from build123d import *

# Parameters (mm, degrees)
ESQUISSE1_W             = 23.5
ESQUISSE1_H             = 23.5
ESQUISSE1_W_2           = 20
ESQUISSE1_H_2           = 20
BOSS_EXTRU_1_DEPTH      = 200
ESQUISSE2_R             = 7.210256751
ENL_V_MAT_EXTRU_1_DEPTH = 1.75


with BuildPart() as part:
    # Esquisse1 → Boss.-Extru.1 (new body)
    with BuildSketch(Plane.XY):
        Rectangle(ESQUISSE1_W, ESQUISSE1_H)
        Rectangle(ESQUISSE1_W_2, ESQUISSE1_H_2, mode=Mode.SUBTRACT)
    extrude(amount=BOSS_EXTRU_1_DEPTH)

    # Esquisse2 → Enlèv. mat.-Extru.1 (cut)
    with BuildSketch(Plane.ZY.offset(11.75)):
        with Locations((100, 0)):
            Circle(ESQUISSE2_R)
    extrude(amount=-ENL_V_MAT_EXTRU_1_DEPTH, mode=Mode.SUBTRACT)


solid = part.part
CAD build for the part. Positions are in the model's coordinates, mm. A direction names the side the tool comes from. Give positions to 0.01 mm unless a question says otherwise; leave off trailing zeros. Write each loop counter-clockwise with the first axis right and the second up, starting at its lowest first coordinate (ties: lowest second). Pieces come first, ordered by that corner, then holes. Notation, with made-up numbers: (18.5, 74) -> (26.5, 74) arc R13 cw to (26.5, 82) -> close; hole circle Ø8 at (-29.75, 42.25). An arc over 180 degrees is marked (long way). Return JSON: item names as keys, results as strings.
Item 1: Tool access for faces 5 (the cylindrical face through (-10.887, 0.317, 92.797)), 6 (the flat face through (10, 0, 99)), 7 (the flat face through (-11, 0, 200)): list every direction of +Z, -Z, +X, -X, +Y, -Y with a clear straight run to the whole face (end or side of a thin tool).
Answer below:
{"face 5": "-X", "face 6": "+Z, -Z", "face 7": "+Z, +X, -X, +Y, -Y"}
Item 2: Band-saw the part on C-C (x = -2). List the corners of the cut face in (y, z), then the cut area to 3 significant figures.
Answer below:
{"outline": "(-11.75, 0) -> (-10, 0) -> (-10, 200) -> (-11.75, 200) -> close; (10, 0) -> (11.75, 0) -> (11.75, 200) -> (10, 200) -> close", "area": "700 mm2"}
Item 3: Drill centre lines: probe 1 along X at (y, z) = (-1.5, 169); probe 2 along Y at (x, z) = (-10.75, 100). Where is each one in solid material? Low to high.
Answer below:
{"probe 1": "x = -11.75 to -10, 10 to 11.75", "probe 2": "y = -11.75 to -7.21, 7.21 to 11.75"}
Item 4: Two-plate mould, pull along Y, no slides. Class faces 1 (the flat face through (11.75, 0, 99)), 2 (the flat face through (0, -10, 99)), 3 (the flat face through (-10, 9, 99)), 4 (the flat face through (0, 11.75, 99)): +Y half, -Y half, draft (parallel to the pull), parting line (faces both ways), or undercut.
Answer below:
{"face 1": "draft", "face 2": "undercut", "face 3": "undercut", "face 4": "+Y half"}
Item 5: Band-saw the part on D-D (z = 100). List the corners of the cut face in (x, y).
Answer below:
{"outline": "(-11.75, -11.75) -> (11.75, -11.75) -> (11.75, 11.75) -> (-11.75, 11.75) -> (-11.75, 7.21) -> (-10, 7.21) -> (-10, 10) -> (10, 10) -> (10, -10) -> (-10, -10) -> (-10, -7.21) -> (-11.75, -7.21) -> close"}
Item 6: Band-saw the part on B-B (z = 20). List the corners of the cut face in (x, y), then the cut area to 3 significant figures.
Answer below:
{"outline": "(-11.75, -11.75) -> (11.75, -11.75) -> (11.75, 11.75) -> (-11.75, 11.75) -> close; hole (-10, -10) -> (10, -10) -> (10, 10) -> (-10, 10) -> close", "area": "152 mm2"}
Item 7: Band-saw the part on A-A (y = 0). List the corners of the cut face in (x, z).
Answer below:
{"outline": "(-11.75, 0) -> (-10, 0) -> (-10, 92.79) -> (-11.75, 92.79) -> close; (-11.75, 107.21) -> (-10, 107.21) -> (-10, 200) -> (-11.75, 200) -> close; (10, 0) -> (11.75, 0) -> (11.75, 200) -> (10, 200) -> close"}
